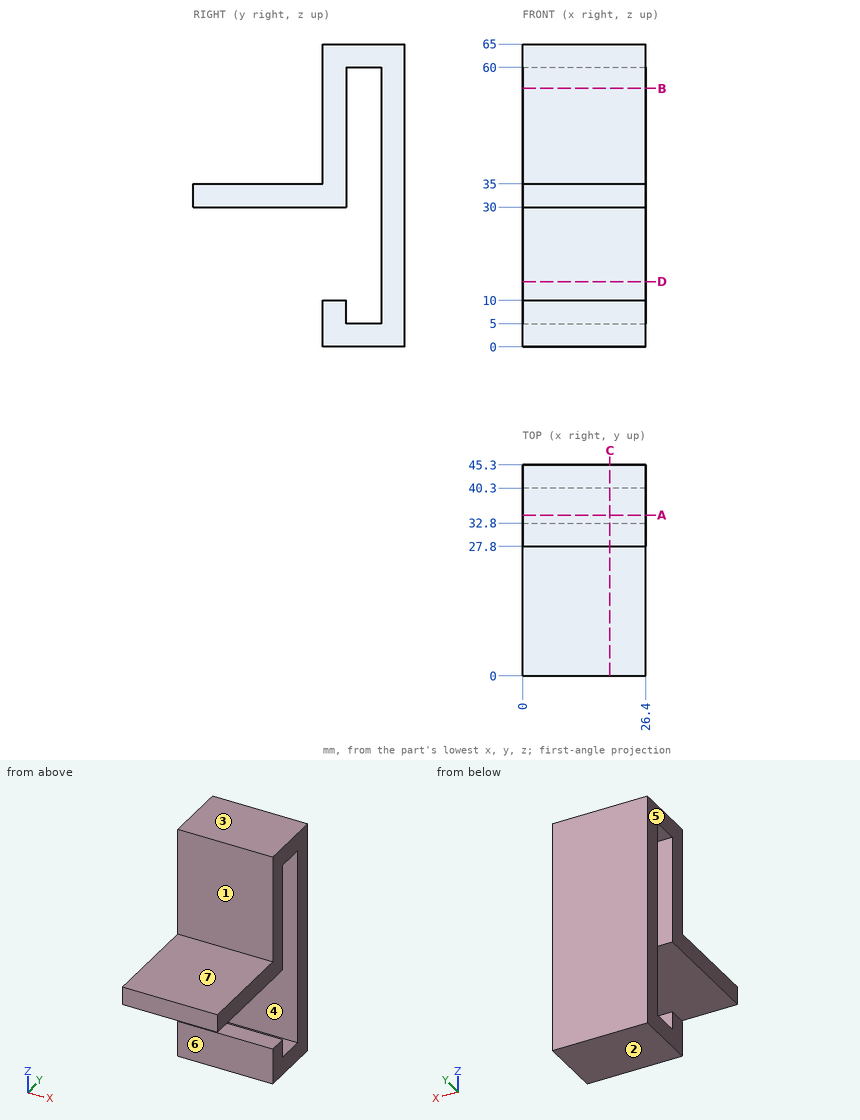
Print and shaded views of the part. All mm, measured from the part's lowest x, y and z. A direction names the side the tool comes from. Round coordinates to 2 decimals unless told otherwise and drop trailing zeros. Write each loop counter-clockwise with the first axis right and the second up, starting at its lowest first coordinate (ties: lowest second). Pieces come first, ordered by that corner, then holes. Notation, with made-up numbers: (-28, 23.25) -> (-2, 23.25) arc R14 ccw to (-2, 29.25) -> close; hole circle Ø10 at (69, 18.5). An arc over 180 degrees is marked (long way). Return JSON: item names as keys, results as strings. Group by question number.
Q1. Saw through at C-C on x = 18.75. Write the cut outline in (y, z).
Q2. Saw through at A-A on y = 34.5. Write the cut outline in (x, z).
Q3. Saw through at B-B on z = 55.5. Write the cut outline in (x, y), plus the area to 3 significant figures.
Q4. Pin check, flat tips, straight feed: pin 1 (13 mm diameter, centred on x = 7.5, z = 54.5, fed in from -Y); pin 2 (1 mm diameter, centred on y = 38.5, z = 18, fed in from -X); pin 3 (8 mm diameter, centred on x = 9, z = 24, fed in from -Y); pin 4 (8 mm diameter, centred on x = 13.5, y = 22, fed in from -Z). Stop position of each tip, or through.
Q5. Which spindle directions (+Z, -Z, +X, -X, +Y, -Y) get a long thin tool onto all of the face, cutting with end or side? Do the marked faces 5, 6 and 7. Say none if no direction does.
Q6. Probe L1, parallel to Y at x = 18.5, z = 50.5; L2, parallel to Z at x = 9.5, y = 37; L3, parallel to Z at x = 6.25, y = 29. List the from-to ranges inside material, lowest first. Write a range as [from, to].
Q7. Saw through at D-D on z = 14. Write the cut outline in (x, y).
Q8. Mould opens along Z. For the marked faces 1, 2, 3 and 4 say: pulls with the +Z half, pulls with the -Z half, needs draft (parallel to the pull), parting line crosses it, or undercut.
Answer:
{
 "1": {"outline": "(0, 30) -> (32.8, 30) -> (32.8, 60) -> (40.3, 60) -> (40.3, 5) -> (32.8, 5) -> (32.8, 10) -> (27.8, 10) -> (27.8, 0) -> (45.3, 0) -> (45.3, 65) -> (27.8, 65) -> (27.8, 35) -> (0, 35) -> close"},
 "2": {"outline": "(0, 0) -> (26.4, 0) -> (26.4, 5) -> (0, 5) -> close; (0, 60) -> (26.4, 60) -> (26.4, 65) -> (0, 65) -> close"},
 "3": {"outline": "(0, 27.8) -> (26.4, 27.8) -> (26.4, 32.8) -> (0, 32.8) -> close; (0, 40.3) -> (26.4, 40.3) -> (26.4, 45.3) -> (0, 45.3) -> close", "area": "264 mm2"},
 "4": {"pin 1": "y = 27.8", "pin 2": "through", "pin 3": "y = 40.3", "pin 4": "z = 30"},
 "5": {"face 5": "+Z, -Z, -X, +Y, -Y", "face 6": "-Z, +X, -X, -Y", "face 7": "+Z, +X, -X, -Y"},
 "6": {"L1": "[27.8, 32.8], [40.3, 45.3]", "L2": "[0, 5], [60, 65]", "L3": "[0, 10], [30, 65]"},
 "7": {"outline": "(0, 40.3) -> (26.4, 40.3) -> (26.4, 45.3) -> (0, 45.3) -> close"},
 "8": {"face 1": "needs draft", "face 2": "pulls with the -Z half", "face 3": "pulls with the +Z half", "face 4": "undercut"}
}
